The listing builds one solid part. Answer for the finished solid, in the listing's coordinates (mm). A direction names the side the tool comes from. Coordinates: 2 decimals unless noted, no trailing zeros. Order: outer loops, then holes, each group sorted by start corner. A loop starts at its lowest first (then second) coordinate and runs counter-clockwise, first axis right, second up.
from build123d import *

# Parameters (mm, degrees)
SKETCH1_W           = 43.5
SKETCH1_H           = 25.25
BOSS_EXTRUDE1_DEPTH = 4
SKETCH5_R           = 10
CUT_EXTRUDE3_DEPTH  = 2
SKETCH6_R           = 12.625
BOSS_EXTRUDE3_DEPTH = 1
SKETCH2_R           = 1.25
CUT_EXTRUDE4_DEPTH  = 26.640848757
SKETCH4_R           = 1.75
BOSS_EXTRUDE2_DEPTH = 4
FILLET1_R           = 2


with BuildPart() as part:
    # Sketch1 → Boss-Extrude1 (new body)
    with BuildSketch(Plane(origin=(0, 0, 0), x_dir=(1, 0, 0), z_dir=(0, 1, 0))):
        Rectangle(SKETCH1_W, SKETCH1_H)
    extrude(amount=BOSS_EXTRUDE1_DEPTH)

    # Sketch5 → Cut-Extrude3 (cut)
    with BuildSketch(Plane(origin=(0, 4, 0), x_dir=(1, 0, 0), z_dir=(0, 1, 0))):
        with Locations(Location((0, 0, 0), (0, 0, 270))):
            Circle(SKETCH5_R)
    extrude(amount=-CUT_EXTRUDE3_DEPTH, mode=Mode.SUBTRACT)

    # Sketch6 → Boss-Extrude3 (add)
    with BuildSketch(Plane.XZ):
        with Locations(Location((0, 0, 0), (0, 0, 270))):
            Circle(SKETCH6_R)
    extrude(amount=BOSS_EXTRUDE3_DEPTH)

    # Sketch2 → Cut-Extrude4 (cut, through all)
    with BuildSketch(Plane(origin=(0, 4, 0), x_dir=(1, 0, 0), z_dir=(0, 1, 0))):
        with Locations(Location((0, 7, 0), (0, 0, 270))):
            Circle(SKETCH2_R)
        with Locations(Location((7, 0, 0), (0, 0, 270))):
            Circle(SKETCH2_R)
        with Locations(Location((0, -7, 0), (0, 0, 270))):
            Circle(SKETCH2_R)
        with Locations(Location((-7, 0, 0), (0, 0, 270))):
            Circle(SKETCH2_R)
    extrude(amount=-CUT_EXTRUDE4_DEPTH, mode=Mode.SUBTRACT)

    # Sketch4 → Boss-Extrude2 (add)
    # profile 1 of 2: a face of its own
    with BuildSketch(Plane.XY.offset(12.625)):
        with BuildLine():
            Line((-21.75, 0), (-15.75, 0))
            Line((-15.75, 0), (-15.75, -3.5))
            ThreePointArc((-15.75, -3.5), (-18.75, -6.5), (-21.75, -3.5))
            Line((-21.75, -3.5), (-21.75, 0))
        make_face()
        with Locations((-18.75, -3.5)):
            Circle(SKETCH4_R, mode=Mode.SUBTRACT)
    # profile 2 of 2: a face of its own
    with BuildSketch(Plane.XY.offset(12.625)):
        with BuildLine():
            Line((21.75, 0), (21.75, -3.5))
            ThreePointArc((21.75, -3.5), (18.75, -6.5), (15.75, -3.5))
            Line((15.75, -3.5), (15.75, 0))
            Line((15.75, 0), (21.75, 0))
        make_face()
        with Locations((18.75, -3.5)):
            Circle(SKETCH4_R, mode=Mode.SUBTRACT)
    boss_extrude2 = extrude(amount=-BOSS_EXTRUDE2_DEPTH)

    # Mirror1: Boss-Extrude2 across plane
    add(boss_extrude2.mirror(Plane.XY))

    # Fillet1
    fillet1_edges = [part.edges().sort_by_distance(p)[0] for p in [
        (-21.75, 4, 0),
        (21.75, 4, 0),
    ]]
    fillet(fillet1_edges, radius=FILLET1_R)


solid = part.part
(1) Given pin 1 Ø3 at (x, z) = (0, -7) entering from +Y; pin 2 Ø1 at (x, z) = (11, 3) entering from -Y, each flat-ended and moving along its own axis, determine where each tip first touches the part or whether it passes through.
(2) Find section D-D on y = -2.5. Count the separate pieces of the cut face and the enclosed holes in it, then the cut area to 3 significant figures.
(3) Find section C-C on y = 1. Determine the outline of the cut face in (x, z) (3 decimals), then the cut area to 3 significant figures.
(4) The mould has two halves that part along Z. Classify faces 1 (the flat face through (0, 2, 0)), 2 (the flat face through (-9, 4, 5)), 3 (the flat face through (0, 1, -12.625)): pulls with the +Z half, pulls with the -Z half, needs draft (parallel to the pull), parting line crosses it, or undercut.
(5) Find section B-B on x = -18.75. Determine the outline of the cut face in (y, z) (3 decimals), then the cut area to 3 significant figures.
(6) Find the intervals of material crossed by probe 1 along X at (y, z) = (1.15, 0); probe 2 along Y at (x, z) = (18.75, -10.6); probe 3 along Y at (x, z) = (0, 9), in increasing order.
(7) A tool of negligible diameter and unlimited length cuts with its end or side. For faces 4 (the cylindrical face through (-7.68, -0.49, 10.02)), 5 (the flat face through (20, -2, 8.625)), 6 (the flat face through (-15.75, -2, -11)), 7 (the cylindrical face through (17.36, -4.56, 10.65)), 8 (the flat face through (-17, -2, -8.625)), from which of +Z, -Z, +X, -X, +Y, -Y can it reach the whole face along a straight path? Write none if from no direction.
(8) Find section A-A on z = 0. Determine the outline of the cut face in (x, y) (3 decimals).
Resolved:
1. pin 1: stops at y = 2
1. pin 2: stops at y = -1
2. separate pieces: 8
2. enclosed holes: 0
2. area: 50.0 mm2
3. outline: (-21.75, -12.625) - (21.75, -12.625) - (21.75, 12.625) - (-21.75, 12.625) - close; hole circle Ø2.5 at (-7, 0); hole circle Ø2.5 at (0, -7); hole circle Ø2.5 at (0, 7); hole circle Ø2.5 at (7, 0)
3. area: 1,080 mm2
4. face 1: undercut
4. face 2: needs draft
4. face 3: pulls with the -Z half
5. outline: (-6.5, -12.625) - (-5.25, -12.625) - (-5.25, -8.625) - (-6.5, -8.625) - close; (-6.5, 8.625) - (-5.25, 8.625) - (-5.25, 12.625) - (-6.5, 12.625) - close; (-1.75, -12.625) - (4, -12.625) - (4, 12.625) - (-1.75, 12.625) - (-1.75, 8.625) - (0, 8.625) - (0, -8.625) - (-1.75, -8.625) - close
5. area: 125 mm2
6. probe 1: x = -21.75 to -8.25, -5.75 to 5.75, 8.25 to 21.75
6. probe 2: y = -6.5 to -5.25, -1.75 to 4
6. probe 3: y = -1 to 2
7. face 4: -Y
7. face 5: +X, -Y
7. face 6: +Z, -Z, -Y
7. face 7: +Z, -Z
7. face 8: -X, -Y
8. outline: (-21.75, 0) - (-12.625, 0) - (-12.625, -1) - (-8.25, -1) - (-8.25, 2) - (-10, 2) - (-10, 4) - (-19.75, 4) arc R2 ccw to (-21.75, 2) - close; (-5.75, -1) - (5.75, -1) - (5.75, 2) - (-5.75, 2) - close; (8.25, -1) - (12.625, -1) - (12.625, 0) - (21.75, 0) - (21.75, 2) arc R2 ccw to (19.75, 4) - (10, 4) - (10, 2) - (8.25, 2) - close
